Autodesk Inventor part; units mm, degrees
ref_plane "YZ Plane" through (0, 0, 0) normal (1, 0, 0) x (0, 1, 0)
ref_plane "XZ Plane" through (0, 0, 0) normal (0, 1, 0) x (-1, 0, 0)
ref_plane "XY Plane" through (0, 0, 0) normal (0, 0, 1) x (1, 0, 0)
sketch "Sketch1" plane through (0, 0, 0) normal (0, 1, 0) x (-1, 0, 0)
  line L0 (99, 99) -> (-99, 99)
  line L1 (-99, 99) -> (-99, -99)
  line L2 (-99, -99) -> (99, -99)
  line L3 (99, -99) -> (99, 99)
  line L4 (99, 99) -> (-99, -99) construction
  line L5 (-99, 99) -> (99, -99) construction
  point P0 (0, 0)
  dimension "d0" = 198
  dimension "d1" = 198
extrude "Box" add sketch "Sketch1" along normal blind 198
sketch "Sketch2" plane through (99, 0, 99) normal (1, 0, 0) x (0, 0, -1)
  point P0 (99, 0)
  point P1 (99, 99)
hole "DecAxisHole" at (99, 99, 0) direction (-1, 0, 0) diameter 66 depth 198
sketch "Sketch3" plane through (0, 0, 0) normal (0, -1, 0) x (1, 0, 0)
  point P0 (0, 0)
  point P1 (-76, -76)
  point P2 (76, -76)
  point P3 (76, 76)
  point P4 (-76, 76)
hole "BoltHoles" at (-76, 0, -76) at (76, 0, -76) at (76, 0, 76) at (-76, 0, 76) direction (0, 1, 0) diameter 8 depth 24 tip angle 118
fillet "Fillet1" radius 1 11 edges at (0, 198, 99) (-99, 198, 0) (99, 198, 0) (99, 99, 99) (-99, 99, 99) (0, 0, 99) (99, 0, 0) (99, 99, -99) (0, 0, -99) (0, 198, -99) (-99, 99, -99)
properties part number "RaDecConnector"
Model file for the job. Use its own axes, mm. A direction names the side the tool comes from. Give positions to 0.01 mm unless a question says otherwise; leave off trailing zeros. Order: outer loops, then holes, each group sorted by start corner. A loop starts at its lowest first (then second) coordinate and runs counter-clockwise, first axis right, second up.
1) Pin check, flat tip, straight feed: pin 1 (7 mm diameter, centred on x = -76, z = 76, fed in from -Y). Stop position of the tip, or through.
2) Saw through at B-B, the plane y = 99. Write the cut outline in (x, z), then the cut area to 3 significant figures.
3) 3-axis set-ups, long thin cutter, end or side, ignore diameter. For faces 1 (the flat face through (-99, 75, -23)), 2 (the cylindrical face through (79.905, 12.168, 76.867)): which of +Z, -Z, +X, -X, +Y, -Y reach the whole face in a straight line?
4) Mould opens along X. For faces 3 (the flat face through (99, 98, -42)), 4 (the flat face through (1, 0, 1)), 5 (the cylindrical face through (-72.095, 12.168, -75.133)) say: +X half, -X half, draft (parallel to the pull), parting line (faces both ways), or undercut.
5) Wall check: probe 1 along Z at (x, y) = (76, 17.5); probe 2 along Y at (x, z) = (9, 0). Give the ranges that are in metal, low to high.
6) Saw through at C-C, the plane y = 126.5. Write the cut outline in (x, z), then the cut area to 3 significant figures.
7) Saw through at A-A, the plane x = 57.5. Write the cut outline in (y, z).
Computed:
1. pin 1: stops at y = 24.3
2. outline: (-99, -98) arc R1 ccw to (-98, -99) - (98, -99) arc R1 ccw to (99, -98) - (99, -33) - (-99, -33) - close; (-99, 33) - (99, 33) - (99, 98) arc R1 ccw to (98, 99) - (-98, 99) arc R1 ccw to (-99, 98) - close
2. area: 26,100 mm2
3. face 1: +Z, -Z, -X, +Y, -Y
3. face 2: -Y
4. face 3: +X half
4. face 4: draft
4. face 5: undercut
5. probe 1: z = -99 to -80, -72 to 72, 80 to 99
5. probe 2: y = 0 to 66, 132 to 198
6. outline: (-99, -98) arc R1 ccw to (-98, -99) - (98, -99) arc R1 ccw to (99, -98) - (99, -18.24) - (-99, -18.24) - close; (-99, 18.24) - (99, 18.24) - (99, 98) arc R1 ccw to (98, 99) - (-98, 99) arc R1 ccw to (-99, 98) - close
6. area: 32,000 mm2
7. outline: (0, -98) arc R1 ccw to (1, -99) - (197, -99) arc R1 ccw to (198, -98) - (198, 98) arc R1 ccw to (197, 99) - (1, 99) arc R1 ccw to (0, 98) - close; hole circle Ø66 at (99, 0)
